from build123d import *

# Parameters (mm, degrees)
SKETCH1_R = 0.25


with BuildPart() as part:
    # Sweep1: sweep along a path in Sketch2
    with BuildLine(Plane.XY) as sweep1_path:
        Line((-2.499404207, 0), (-2.499404207, 16))
        ThreePointArc((-2.499404207, 16), (-1.913617769, 17.414213562), (-0.499404207, 18))
        Line((-0.499404207, 18), (0.500595793, 18))
        ThreePointArc((0.500595793, 18), (1.914809356, 17.414213562), (2.500595793, 16))
        Line((2.500595793, 16), (2.500595793, 0))
    # Sketch1 → Sweep1 (sweep)
    with BuildSketch(Plane(origin=(0, 0, 0), x_dir=(1, 0, 0), z_dir=(0, 1, 0))):
        with Locations((-2.499404207, 0)):
            Circle(SKETCH1_R)
    sweep(path=sweep1_path.line)


solid = part.part
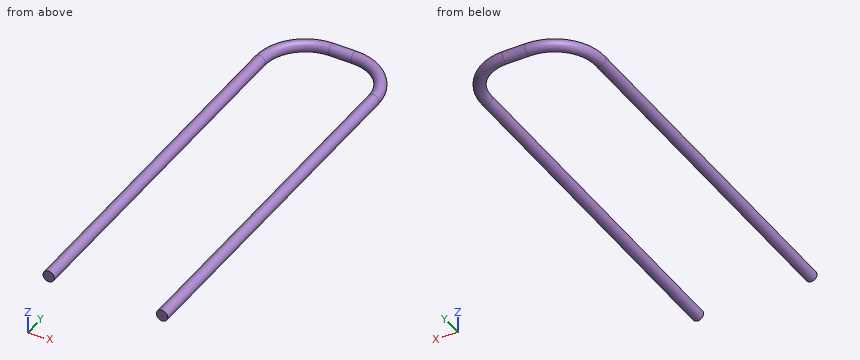
Design review of the part built by this model. Coordinates are the model's own, in mm. Round coordinates to 2 decimals unless told otherwise and drop trailing zeros. Loops run counter-clockwise (first coordinate to the right, second up) from the corner with the lowest first, then second, coordinate; pieces in that order, holes last. Notation, with made-up numbers: (21, -35.75) -> (44, -35.75) arc R27 ccw to (44, 1.25) -> close; hole circle Ø11 at (86.25, 56). An arc over 180 degrees is marked (long way). Use one line per item in the form item = value. Start each with the question number.
Q1. Wall thickness on line 1 along X through (y, z) = (11.75, 0); line 2 along X through (y, z) = (12.75, -0.05); line 3 along Y through (x, z) = (-0.5, 0): over which ranges is each line inside the solid? List them lowest first. Write a range as [from, to].
Q2. We need section B-B on y = 11.75. Give the boundary of the cut face in (x, z).
Q3. For pin 1 Ø2 at (x, y) = (-2, 16.5) entering from +Z, flat-tipped, find the tip position at first contact; note if it passes through.
Q4. We need section A-A on z = 0. Give the boundary of the cut face in (x, y).
Calculated:
q1.line_1 = [-2.75, -2.25], [2.25, 2.75]
q1.line_2 = [-2.74, -2.25], [2.26, 2.75]
q1.line_3 = [17.75, 18.25]
q2.outline = circle Ø0.5 at (-2.5, 0); circle Ø0.5 at (2.5, 0)
q3.pin_1 = 0.25
q4.outline = (-2.75, 0) -> (-2.25, 0) -> (-2.25, 16) arc R1.75 cw to (-0.5, 17.75) -> (0.5, 17.75) arc R1.75 cw to (2.25, 16) -> (2.25, 0) -> (2.75, 0) -> (2.75, 16) arc R2.25 ccw to (0.5, 18.25) -> (-0.5, 18.25) arc R2.25 ccw to (-2.75, 16) -> close
